The model under review builds one solid part; all positions refer to its coordinate system, in mm. Give positions to 0.01 mm unless a question says otherwise; leave off trailing zeros. Loops run counter-clockwise (first coordinate to the right, second up) from the corner with the lowest first, then second, coordinate; pieces in that order, holes last. Notation, with made-up numbers: M 10.25,62 L 66.25,62 A13 cw 66.25,85 Z; hole C -7.75,34.5 d1. An arc over 180 degrees is marked long. Write item = value, one per line. Start each with the question number.
1. We need section D-D on y = -25. Give the boundary of the cut face in (x, z).
2. We need section A-A on x = 0. Give the boundary of the cut face in (y, z).
3. We need section C-C on y = -13.5. Give the boundary of the cut face in (x, z), then the cut area to 3 significant figures.
4. We need section B-B on z = 2.1. Give the boundary of the cut face in (x, y).
5. Wall thickness on line 1 along X through (y, z) = (28, 1.2); line 2 along Y through (x, z) = (4.5, 0.7); line 3 along Y through (x, z) = (0, 1.45): over which ranges is each line inside the solid? List them lowest first. Write a range as from..to.
6. For pin 1 (6 mm diameter, centred on x = 25, y = 28, fed in from +Z); pin 2 (3 mm diameter, centred on x = 25, y = -25, fed in from +Z), all flat-tipped, find the tip position at first contact; note any pin that passes through.
7. Draft analysis for pull direction Y (two halves, no side actions). For faces 1 (the face through (20, 16, 3)), 2 (the face through (24.459, -26.717, 0.76)), 3 (the face through (7, 31, 1)), state which applies: pulls with the +Y half, pulls with the -Y half, needs draft (parallel to the pull), parting line crosses it, or undercut.
from build123d import *

# Parameters (mm, degrees)
SKETCH_1_W                  = 60
SKETCH_1_H                  = 62
SKETCH_1_R                  = 26
SKETCH_1_R_2                = 1.6
EXTRUDE_1_DEPTH             = 3
CUT_EXTRUDE_1_DEPTH         = 44.243496621
CUT_EXTRUDE_2_REACH         = 45.243
SKETCH_5_R                  = 1.6
CUT_EXTRUDE_3_DEPTH         = 44.243496621
HOLE_WIZARD_M3_1_AT_2_COUNT = 2
HOLE_WIZARD_M3_1_AT_2_PITCH = 20
HOLE_WIZARD_M3_1_AT_3_COUNT = 2
HOLE_WIZARD_M3_1_AT_3_PITCH = 56.648036153


with BuildPart() as part:
    # 草图1 → 凸台-拉伸1 (new body)
    with BuildSketch(Plane.XY):
        Rectangle(SKETCH_1_W, SKETCH_1_H)
        with Locations((0, -1.5)):
            Circle(SKETCH_1_R, mode=Mode.SUBTRACT)
        with Locations((25, 28)):
            Circle(SKETCH_1_R_2, mode=Mode.SUBTRACT)
        with Locations((5, 28)):
            Circle(SKETCH_1_R_2, mode=Mode.SUBTRACT)
    extrude(amount=EXTRUDE_1_DEPTH)

    # 草图2 → 切除-拉伸1 (cut, through all)
    with BuildSketch(Plane.XY.offset(3)):
        Polygon((-30, 13.123696111), (-15, 31), (-30, 31), align=None)
    extrude(amount=-CUT_EXTRUDE_1_DEPTH, mode=Mode.SUBTRACT)

    # 草图4 → 切除-拉伸2 (cut, up to next)
    with BuildSketch(Plane.XY.offset(3), mode=Mode.PRIVATE) as cut_extrude_2_sk1:
        Polygon((-30, -16), (-15, -31), (-30, -31), align=None)
    cut_extrude_2_tool1 = extrude(cut_extrude_2_sk1.sketch, amount=-CUT_EXTRUDE_2_REACH, mode=Mode.PRIVATE) & part.part
    add(cut_extrude_2_tool1.solids().sort_by_distance((-25, -26, 3))[0], mode=Mode.SUBTRACT)

    # 草图5 → 切除-拉伸3 (cut, through all)
    with BuildSketch(Plane.XY.offset(3)):
        with Locations((25, -25)):
            Circle(SKETCH_5_R)
    extrude(amount=-CUT_EXTRUDE_3_DEPTH, mode=Mode.SUBTRACT)

    # 草图7 → M3 十字槽半沉头木螺钉的锥形沉头孔1 (revolve, cut)
    with BuildSketch(Plane(origin=(5, 28, 3), x_dir=(0, -1, 0), z_dir=(1, 0, 0))):
        Polygon((0, 0), (0, 3), (1.8, 3), (1.8, 1.5), (3.3, 0), align=None)
    hole_wizard_m3_1 = revolve(axis=Axis((5, 28, 9.35), (0, 0, -1)), mode=Mode.SUBTRACT)

    # M3 十字槽半沉头木螺钉的锥形沉头孔1 at 2: M3 十字槽半沉头木螺钉的锥形沉头孔1 ×2
    with Locations(*[(i * HOLE_WIZARD_M3_1_AT_2_PITCH, 0, 0) for i in range(1, HOLE_WIZARD_M3_1_AT_2_COUNT)]):
        add(hole_wizard_m3_1, mode=Mode.SUBTRACT)

    # M3 十字槽半沉头木螺钉的锥形沉头孔1 at 3: M3 十字槽半沉头木螺钉的锥形沉头孔1 ×2
    with Locations(*[Vector(0.35305725243424246, -0.9356017189507422, 0) * (i * HOLE_WIZARD_M3_1_AT_3_PITCH) for i in range(1, HOLE_WIZARD_M3_1_AT_3_COUNT)]):
        add(hole_wizard_m3_1, mode=Mode.SUBTRACT)


solid = part.part
Final values:
q1.outline = M -21,0 L -11.12,0 L -11.12,3 L -21,3 Z; M 11.12,0 L 23.2,0 L 23.2,1.5 L 21.7,3 L 11.12,3 Z; M 26.8,0 L 30,0 L 30,3 L 28.3,3 L 26.8,1.5 Z
q2.outline = M -31,0 L -27.5,0 L -27.5,3 L -31,3 Z; M 24.5,0 L 31,0 L 31,3 L 24.5,3 Z
q3.outline = M -30,0 L -23.07,0 L -23.07,3 L -30,3 Z; M 23.07,0 L 30,0 L 30,3 L 23.07,3 Z
q3.area = 41.6 mm²
q4.outline = M -30,-16 L -15,-31 L 30,-31 L 30,31 L -15,31 L -30,13.12 Z; hole C 0,-1.5 d52; hole C 5,28 d4.8; hole C 25,-25 d4.8; hole C 25,28 d4.8
q5.line_1 = -17.52..3.2, 6.8..23.2, 26.8..30
q5.line_2 = -31..-27.11, 24.11..26.27, 29.73..31
q5.line_3 = -31..-27.5, 24.5..31
q6.pin_1 = 2.7
q6.pin_2 = through
q7.face_1 = needs draft
q7.face_2 = undercut
q7.face_3 = pulls with the +Y half
